Geometry: final body of the model. Coordinates: model frame, mm. A direction names the side the tool comes from. Round coordinates to 2 decimals unless told otherwise and drop trailing zeros. Loops run counter-clockwise (first coordinate to the right, second up) from the corner with the lowest first, then second, coordinate; pieces in that order, holes last. Notation, with made-up numbers: (72.5, -36) - (128.5, -36) arc R21 ccw to (128.5, 0) - close; hole circle Ø8 at (72.25, 88.25). An arc over 180 degrees is marked (long way). Write item = value, one per line. Start each with the question number.
Item 1: Access query for faces 1 (the flat face through (0, -12.7, 17)), 2 (the flat face through (-27.94, -16, 15)), 3 (the flat face through (27.94, 170, 16)). Directions: +Z, -Z, +X, -X, +Y, -Y. A direction counts if a zero-diameter tool reaches every point of the face in a straight line with its end or side. Return the directions, or none.
Item 2: Section B-B (y = 44). Return loops of the section in (x, z) (3 decimals).
Item 3: First-contact query: pin 1 (12 mm diameter, centred on y = 149.5, z = 14, fed in from +X); pin 2 (1.3 mm diameter, centred on y = 178.5, z = 5.5, fed in from +X); pin 3 (4 mm diameter, centred on x = -31.5, y = 113, fed in from +Z). Flat tips, straight axial feed; report the tip coordinate or a pass-through.
Item 4: Section A-A (x = -21). Return loops of the section in (y, z).
Item 5: Line query: line 1 (Z direction, x = 20.5, y = 156.5); line 2 (Y direction, x = 21.5, z = 6); line 3 (Y direction, x = -2.5, z = 19). Output: solid intervals per line, ascending. Write a range as from..to.
Item 6: Draft query along Z for faces 4 (the flat face through (-27.94, 170, 16)), 5 (the flat face through (0, 177.8, 6)), 6 (the cylindrical face through (-46.355, 75.78, 6.261)). Return one class per face: pulls with the +Z half, pulls with the -Z half, needs draft (parallel to the pull), parting line crosses it, or undercut.
from build123d import *

# Parameters (mm, degrees)
SKETCH1_W               = 99.06
SKETCH1_H               = 360.68
BOSS_EXTRUDE1_DEPTH     = 12.7
SKETCH3_W               = 32.004
SKETCH3_H               = 11.43
BOSS_EXTRUDE3_DEPTH     = 20.32
SKETCH2_W               = 55.88
SKETCH2_H               = 12.7
BOSS_EXTRUDE4_DEPTH     = 7.62
CUT_EXTRUDE2_DEPTH      = 38.1
SKETCH6_W               = 50.8
SKETCH6_H               = 5.08
CUT_EXTRUDE3_DEPTH      = 2.54
SKETCH7_R               = 50.8
SKETCH7_R_2             = 46.355
CUT_EXTRUDE4_DEPTH      = 366.559302576
CUT_EXTRUDE5_DEPTH      = 190.107435139
CUT_EXTRUDE5_DEPTH_BACK = 190.107435139
SKETCH8_W               = 158.320369358
SKETCH8_H               = 163.138922325


with BuildPart() as part:
    # Sketch1 → Boss-Extrude1 (new body)
    with BuildSketch(Plane.XY):
        Rectangle(SKETCH1_W, SKETCH1_H)
    extrude(amount=BOSS_EXTRUDE1_DEPTH)

    # Sketch3 → Boss-Extrude3 (add)
    with BuildSketch(Plane(origin=(0, 0, 0), x_dir=(-1, 0, 0), z_dir=(0, 0, -1))):
        with Locations((0, -43.815)):
            Rectangle(SKETCH3_W, SKETCH3_H)
        with Locations((0, -159.385)):
            Rectangle(SKETCH3_W, SKETCH3_H)
    boss_extrude3 = extrude(amount=BOSS_EXTRUDE3_DEPTH)

    # Sketch2 → Boss-Extrude4 (add, symmetric)
    with BuildSketch(Plane.XY.offset(12.7)):
        with Locations((0, 171.45)):
            Rectangle(SKETCH2_W, SKETCH2_H)
        with Locations((0, -19.05)):
            Rectangle(SKETCH2_W, SKETCH2_H)
    extrude(amount=BOSS_EXTRUDE4_DEPTH, both=True)

    # Mirror1: Boss-Extrude3 across plane
    add(boss_extrude3.mirror(Plane.XY.offset(6.35)))

    # Sketch5 → Cut-Extrude2 (cut, symmetric)
    with BuildSketch(Plane(origin=(0, 0, 0), x_dir=(0, 0, -1), z_dir=(1, 0, 0))):
        Polygon((20.32, -153.67), (0, -165.1), (20.32, -165.1), align=None)
        Polygon((-33.02, -153.67), (-12.7, -165.1), (-33.02, -165.1), align=None)
        Polygon((-33.02, -49.53), (-33.02, -38.1), (-12.7, -38.1), align=None)
        Polygon((20.32, -49.53), (0, -38.1), (20.32, -38.1), align=None)
        Polygon((-12.7, 177.8), (-20.32, 165.1), (-20.32, 177.8), align=None)
        Polygon((-20.32, -12.7), (-12.7, -25.4), (-20.32, -25.4), align=None)
    extrude(amount=CUT_EXTRUDE2_DEPTH, both=True, mode=Mode.SUBTRACT)

    # Sketch6 → Cut-Extrude3 (cut)
    with BuildSketch(Plane(origin=(0, 180.34, 0), x_dir=(1, 0, 0), z_dir=(0, 1, 0))):
        with Locations((0, -6.35)):
            Rectangle(SKETCH6_W, SKETCH6_H)
    cut_extrude3 = extrude(amount=-CUT_EXTRUDE3_DEPTH, mode=Mode.SUBTRACT)

    # Mirror2: Cut-Extrude3 across plane
    add(cut_extrude3.mirror(Plane.ZX), mode=Mode.SUBTRACT)

    # Sketch7 → Cut-Extrude4 (cut, through all)
    with BuildSketch(Plane(origin=(0, 180.34, 0), x_dir=(1, 0, 0), z_dir=(0, 1, 0))):
        with Locations((0, -6.35)):
            Circle(SKETCH7_R)
        with Locations((0, -6.35)):
            Circle(SKETCH7_R_2, mode=Mode.SUBTRACT)
    extrude(amount=-CUT_EXTRUDE4_DEPTH, mode=Mode.SUBTRACT)

    # Sketch8 → Cut-Extrude5 (cut, two sides: drawn at the far end of the back side and taken through both)
    with BuildSketch(Plane.XY.offset(-CUT_EXTRUDE5_DEPTH_BACK)):
        with Locations((0.168785042, -113.319461163)):
            Rectangle(SKETCH8_W, SKETCH8_H)
    extrude(amount=CUT_EXTRUDE5_DEPTH + CUT_EXTRUDE5_DEPTH_BACK, mode=Mode.SUBTRACT)


solid = part.part
Taken from the geometry:
q1.face_1 = +Z, +X, -X
q1.face_2 = +Z, -X, +Y, -Y
q1.face_3 = +Z, +X, +Y, -Y
q2.outline = (-45.918, 0) - (45.918, 0) arc R46.355 ccw to (45.918, 12.7) - (-45.918, 12.7) arc R46.355 ccw to start
q3.pin_1 = 46.33
q3.pin_2 = 46.35
q3.pin_3 = 12.7
q4.outline = (-31.75, 0) - (180.34, 0) - (180.34, 3.81) - (177.8, 3.81) - (177.8, 8.89) - (180.34, 8.89) - (180.34, 12.7) - (177.8, 12.7) - (165.1, 20.32) - (165.1, 12.7) - (-12.7, 12.7) - (-12.7, 20.32) - (-25.4, 12.7) - (-31.75, 12.7) - close
q5.line_1 = 0..12.7
q5.line_2 = -31.75..177.8
q5.line_3 = -14.9..-12.7, 165.1..167.3
q6.face_4 = needs draft
q6.face_5 = undercut
q6.face_6 = parting line crosses it
